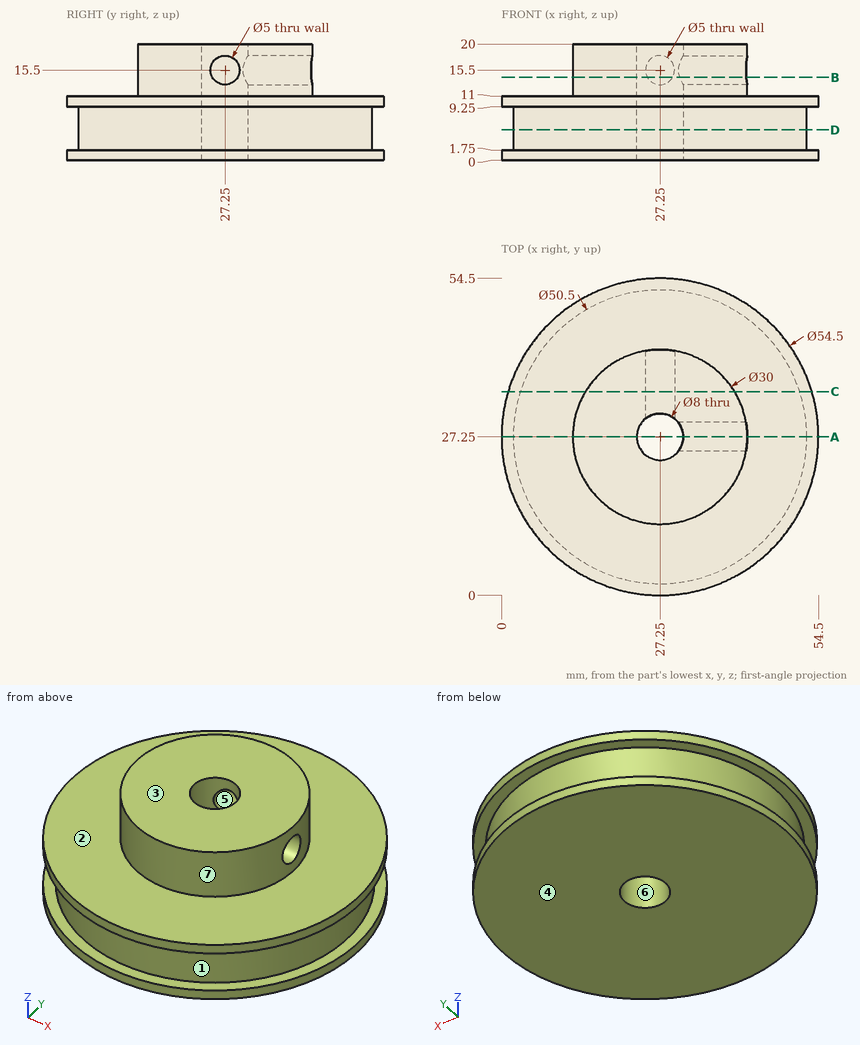
Check sheet for the drawn part. Datum: minimum x, y, z corner. Units: mm. A direction names the side the tool comes from. Round coordinates to 2 decimals unless told otherwise and drop trailing zeros. Loops run counter-clockwise (first coordinate to the right, second up) from the corner with the lowest first, then second, coordinate; pieces in that order, holes last. Notation, with made-up numbers: (10.25, -36.5) - (64.25, -36.5) arc R27 cw to (64.25, -18.5) - close; hole circle Ø4 at (73, -24). An arc over 180 degrees is marked (long way). Write item = value, one per line. Start each with the question number.
1. Thickness scan on line 1 (Z direction, x = 35, y = 27); line 2 (Z direction, x = 8, y = 38); line 3 (X direction, y = 36.25, z = 15.5). Record the ranges inside material, lowest first.
2. Depth check by flat-ended pin: pin 1 (4.5 mm diameter, centred on x = 27.25, z = 15.5, fed in from +Y); pin 2 (2 mm diameter, centred on y = 44, z = 14.5, fed in from -X); pin 3 (3 mm diameter, centred on y = 27.25, z = 15.5, fed in from -X); pin 4 (8 mm diameter, centred on y = 17.5, z = 4, fed in from -X). Enter the tip coordinate at first touch or a pass-through.
3. Mould release check, pull along X, two halves, no side actions. Record for the marked faces 4, 5, 6 and 7: released by +X, released by -X, zero draft, split by the parting line, or undercut.
4. Set-up check for the marked faces 1, 2 and 3: record each of +Z, -Z, +X, -X, +Y, -Y from which the full face is reachable in a straight line by a thin tool's end or side.
5. Section check B-B on z = 14.25. Enter the section's corners in (x, y).
6. Section check C-C on y = 35. Enter the section's corners in (x, z), then the cut area to 3 significant figures.
7. Section check A-A on y = 27.25. Enter the section's corners in (x, z), then the cut area to 4 significant figures.
8. Section check D-D on z = 5.25. Enter the section's corners in (x, y).
Working result:
q1.line_1 = 0 to 13.01, 17.99 to 20
q1.line_2 = 0 to 11
q1.line_3 = 15.25 to 24.75, 29.75 to 39.25
q2.pin_1 = 23.94
q2.pin_2 = through
q2.pin_3 = 12.25
q2.pin_4 = 0.77
q3.face_4 = zero draft
q3.face_5 = undercut
q3.face_6 = undercut
q3.face_7 = split by the parting line
q4.face_1 = none
q4.face_2 = +Z
q4.face_3 = +Z, +X, -X, +Y, -Y
q5.outline = (25.08, 30.61) - (25.08, 42.09) arc R15 ccw (long way) to (42.09, 25.08) - (30.61, 25.08) arc R4 cw (long way) to start; (29.42, 30.61) arc R4 cw to (30.61, 29.42) - (42.09, 29.42) arc R15 ccw to (29.42, 42.09) - close
q6.outline = (1.13, 0) - (53.37, 0) - (53.37, 1.75) - (51.28, 1.75) - (51.28, 9.25) - (53.37, 9.25) - (53.37, 11) - (40.09, 11) - (40.09, 20) - (14.41, 20) - (14.41, 11) - (1.13, 11) - (1.13, 9.25) - (3.22, 9.25) - (3.22, 1.75) - (1.13, 1.75) - close; hole circle Ø5 at (27.25, 15.5)
q6.area = 755 mm^2
q7.outline = (0, 0) - (23.25, 0) - (23.25, 20) - (12.25, 20) - (12.25, 11) - (0, 11) - (0, 9.25) - (2, 9.25) - (2, 1.75) - (0, 1.75) - close; (31.25, 0) - (54.5, 0) - (54.5, 1.75) - (52.5, 1.75) - (52.5, 9.25) - (54.5, 9.25) - (54.5, 11) - (42.25, 11) - (42.25, 13) - (31.25, 13) - close; (31.25, 18) - (42.25, 18) - (42.25, 20) - (31.25, 20) - close
q7.area = 624.5 mm^2
q8.outline = circle Ø50.5 at (27.25, 27.25); hole circle Ø8 at (27.25, 27.25)
